Build history of the part. All positions in model axes, mm. Round coordinates to 2 decimals unless told otherwise and drop trailing zeros. Order: outer loops, then holes, each group sorted by start corner. A loop starts at its lowest first (then second) coordinate and runs counter-clockwise, first axis right, second up. Notation, with made-up numbers: (56.25, 4.5) -> (104.25, 4.5) arc R18 cw to (104.25, 22.5) -> close; hole circle Ø3 at (-1, 87.5). An arc over 180 degrees is marked (long way). Write item = value, one per line.
Autodesk Inventor part; units mm, degrees
ref_plane "工作平面1" through (0, 0, 0) normal (0, 0, 1) x (1, 0, 0)
ref_plane "工作平面2" through (173.2, -616.2, 0) normal (1, 0, 0) x (0, 0, -1)
ref_plane "工作平面3" through (318, -1163.6, 0) normal (1, 0, 0) x (0, 0, -1)
ref_plane "工作平面1" through (0, 0, 0) normal (0, 0, 1) x (1, 0, 0)
sketch "草图1" plane through (0, 0, 0) normal (0, 0, 1) x (1, 0, 0)
  line L0 (0, 0) -> (60, 0)
  line L1 (60, 0) -> (60, -1169.8)
  line L2 (60, -1169.8) -> (0, -1169.8)
  line L3 (0, -1169.8) -> (0, 0)
  line L4 (0, -80.6) -> (60, -80.6)
  line L5 (0, -191.9) -> (60, -191.9)
  line L6 (0, -276.5) -> (60, -276.5)
  line L7 (0, -335.9) -> (60, -335.9)
  line L8 (0, -420.6) -> (60, -420.6)
  line L9 (0, -550.6) -> (60, -550.6)
  line L10 (0, -677.8) -> (60, -677.8)
  line L11 (0, -782.9) -> (60, -782.9)
  line L12 (0, -839.5) -> (60, -839.5)
  line L13 (0, -923.6) -> (60, -923.6)
  line L14 (0, -1007.7) -> (60, -1007.7)
  line L15 (0, -1091.2) -> (60, -1091.2)
  line L16 (60, 0) -> (118.4, 0)
  line L17 (118.4, 0) -> (118.4, -23.7)
  line L18 (118.4, -23.7) -> (83.4, -23.7)
  line L19 (83.4, -23.7) -> (83.4, -79.7)
  line L20 (83.4, -79.7) -> (118.4, -79.7)
  line L21 (118.4, -79.7) -> (118.4, -137.6)
  line L22 (118.4, -137.6) -> (83.4, -137.6)
  line L23 (83.4, -137.6) -> (83.4, -276.5)
  line L24 (83.4, -276.5) -> (142.9, -276.5)
  line L25 (142.9, -276.5) -> (142.9, -379.5)
  line L26 (83.4, -276.5) -> (83.4, -379.5)
  line L27 (83.4, -379.5) -> (142.9, -379.5)
  line L28 (142.9, -379.5) -> (142.9, -463)
  line L29 (142.9, -463) -> (83.4, -463)
  line L30 (83.4, -463) -> (83.4, -379.5)
  line L31 (142.9, -463) -> (142.9, -566.2)
  line L32 (142.9, -566.2) -> (83.4, -566.2)
  line L33 (83.4, -566.2) -> (83.4, -463)
  line L34 (142.9, -566.2) -> (146.7, -566.2)
  line L35 (146.7, -566.2) -> (146.7, -616.2)
  line L36 (146.7, -616.2) -> (192.5, -616.2)
  line L37 (192.5, -616.2) -> (192.5, -673.2)
  line L38 (192.5, -616.2) -> (342.5, -616.2)
  line L39 (342.5, -616.2) -> (342.5, -673.2)
  line L40 (342.5, -673.2) -> (143.4, -673.2)
  line L41 (143.4, -673.2) -> (83.4, -673.2)
  line L42 (83.4, -673.2) -> (83.4, -1092.3)
  line L43 (83.4, -1092.3) -> (143.4, -1092.3)
  line L44 (143.4, -1092.3) -> (143.4, -673.2)
  line L45 (83.4, -754.3) -> (143.4, -754.3)
  line L46 (143.4, -837.8) -> (83.4, -837.8)
  line L47 (83.4, -893.6) -> (143.4, -893.6)
  line L48 (143.4, -978.3) -> (83.4, -978.3)
  line L49 (60, -1169.8) -> (188.1, -1169.8)
  line L50 (188.1, -1169.8) -> (188.1, -1092.3)
  line L51 (188.1, -1092.3) -> (143.4, -1092.3)
  line L52 (83.4, -1092.3) -> (83.4, -1117.3)
  line L53 (83.4, -1117.3) -> (188.1, -1117.3)
  line L54 (98.6, -1092.3) -> (98.6, -1117.3)
  line L55 (114.5, -1092.3) -> (114.5, -1117.3)
  line L56 (143.4, -1092.3) -> (143.4, -1117.3)
  line L57 (166.2, -1092.3) -> (166.2, -1117.3)
  line L58 (188.1, -1163.6) -> (336, -1163.6)
  line L59 (188.1, -1137.1) -> (336, -1137.1)
  line L60 (336, -1137.1) -> (336, -1163.6)
  dimension "d1" = 60
  dimension "d2" = 80.6
  dimension "d3" = 111.3
  dimension "d4" = 84.6
  dimension "d5" = 59.4
  dimension "d6" = 84.7
  dimension "d7" = 130
  dimension "d8" = 127.2
  dimension "d9" = 105.1
  dimension "d10" = 56.6
  dimension "d11" = 84.1
  dimension "d12" = 84.1
  dimension "d13" = 83.5
  dimension "d14" = 78.6
  dimension "d15" = 58.4
  dimension "d16" = 23.7
  dimension "d17" = 35
  dimension "d18" = 56
  dimension "d19" = 57.9
  dimension "d20" = 35
  dimension "d21" = 138.9
  dimension "d22" = 59.5
  dimension "d23" = 103
  dimension "d24" = 83.5
  dimension "d25" = 103.2
  dimension "d26" = 59.5
  dimension "d27" = 3.8
  dimension "d28" = 50
  dimension "d29" = 45.8
  dimension "d30" = 57
  dimension "d31" = 150
  dimension "d32" = 57
  dimension "d33" = 199.1
  dimension "d34" = 60
  dimension "d36" = 81.1
  dimension "d37" = 83.5
  dimension "d38" = 55.8
  dimension "d39" = 84.7
  dimension "d40" = 114
  dimension "d41" = 128.1
  dimension "d42" = 25
  dimension "d43" = 15.2
  dimension "d44" = 15.9
  dimension "d45" = 28.9
  dimension "d46" = 22.8
  dimension "d47" = 21.9
  dimension "d48" = 147.9
  dimension "d49" = 6.2
  dimension "d50" = 26.5
extrude "拉伸1" add sketch "草图1" against normal blind 1
sketch "草图2" plane through (0, 0, 0) normal (0, 0, 1) x (1, 0, 0)
  line L0 (342.5, -616.2) -> (146.7, -616.2) construction
  line L1 (342.5, -673.2) -> (342.5, -616.2) construction
  line L2 (143.4, -673.2) -> (342.5, -673.2) construction
  line L3 (146.7, -616.2) -> (146.7, -566.2) construction
  line L4 (150.3, -616.2) -> (150.3, -596.9)
  line L5 (150.3, -596.9) -> (196.1, -596.9)
  line L6 (196.1, -596.9) -> (196.1, -616.2)
  line L7 (150.3, -616.2) -> (196.1, -616.2)
  point P0 (0, 0)
  dimension "d53" = 19.3
  dimension "d54" = 45.8
  dimension "d55" = 3.6
extrude "拉伸2" add sketch "草图2" against normal up to surface (1 mm away)
ref_plane "工作平面2" through (173.2, -616.2, 0) normal (1, 0, 0) x (0, 0, -1)
sketch "草图3" plane through (173.2, -616.2, 0) normal (1, 0, 0) x (0, 0, -1)
  line L0 (0, 19.3) -> (1, 19.3) construction
  line L1 (0.5, 19.3) -> (-20.5, 61.3)
  line L2 (0.5, 19.3) -> (0.1, 19.3)
  line L3 (0.1, 19.3) -> (-20.9, 61.3)
  line L4 (-20.9, 61.3) -> (-20.5, 61.3)
  line L5 (-20.9, 61.3) -> (-20.9, 83.8)
  line L6 (-20.9, 83.8) -> (-20.5, 83.8)
  line L7 (-20.5, 83.8) -> (-20.5, 61.3)
  point P0 (0, 616.2)
  dimension "d58" = 42
  dimension "d60" = 21
  dimension "d61" = 0.4
  dimension "d64" = 22.5
extrude "拉伸3" add sketch "草图3" along normal up to surface (22.9 mm away)
extrude "拉伸4" add sketch "草图3" against normal up to surface (22.9 mm away) contours L4 L5 L6 L7
sketch "草图5" plane through (150.3, -554.9, 20.5) normal (-1, 0, 0) x (0, 0, 1)
  line L0 (0.4, 0) -> (0, 0) construction
  line L1 (0.2, 0) -> (21.2, -42) construction
  line L2 (0, 0) -> (21, -42)
  line L3 (0.4, 0) -> (0, 0)
  line L4 (0.4, 0) -> (21.4, -42)
  line L5 (21.4, -42) -> (21.2, -42)
  line L6 (21, -42) -> (21.2, -42)
  line L7 (21.4, -42) -> (21.4, -61.3)
  line L8 (21.4, -61.3) -> (21, -61.3)
  line L9 (21, -61.3) -> (21, -42)
  point P0 (-20.5, 554.9)
  dimension "d67" = 42
  dimension "d69" = 21
  dimension "d71" = 19.3
extrude "拉伸5" add sketch "草图5" against normal up to surface (22.9 mm away)
ref_plane "工作平面3" through (318, -1163.6, 0) normal (1, 0, 0) x (0, 0, -1)
sketch "草图6" plane through (318, -1163.6, 0) normal (1, 0, 0) x (0, 0, -1)
  line L0 (0, 26.5) -> (1, 26.5) construction
  line L1 (0.5, 26.5) -> (-20.5, 68.5)
  line L2 (0.5, 26.5) -> (0.1, 26.5)
  line L3 (0.1, 26.5) -> (-20.9, 68.5)
  line L4 (-20.9, 68.5) -> (-20.5, 68.5)
  line L5 (-20.9, 68.5) -> (-20.9, 93.5)
  line L6 (-20.9, 93.5) -> (-20.5, 93.5)
  line L7 (-20.5, 93.5) -> (-20.5, 68.5)
  point P0 (0, 1163.6)
  dimension "d75" = 42
  dimension "d77" = 21
  dimension "d78" = 0.4
  dimension "d79" = 25
  dimension "d80" = 0.4
extrude "拉伸6" add sketch "草图6" against normal blind 40
sketch "草图7" plane through (318, -1163.6, 0) normal (1, 0, 0) x (0, 0, -1)
  line L0 (-20.9, 93.5) -> (-20.9, 68.5) construction
  line L1 (-20.5, 68.5) -> (-20.5, 93.5) construction
  line L2 (-20.5, 93.5) -> (-20.9, 93.5) construction
  line L3 (-20.9, 93.5) -> (-20.5, 93.5)
  line L4 (-20.5, 93.5) -> (-20.5, 68.5)
  line L5 (-20.5, 68.5) -> (-20.9, 68.5)
  line L6 (-20.9, 68.5) -> (-20.9, 93.5)
  line L7 (-20.5, 68.5) -> (-41.5, 26.5)
  line L8 (-20.9, 68.5) -> (-41.9, 26.5)
  line L9 (-41.9, 26.5) -> (-41.5, 26.5)
  point P0 (0, 1163.6)
  dimension "d83" = 21
  dimension "d84" = 42
extrude "拉伸7" add sketch "草图7" along normal up to surface (18 mm away)
ref_plane "工作平面4" through (298, -1163.6, 0) normal (1, 0, 0) x (0, 0, -1)
mirror "镜像1" about plane through (298, -1163.6, 0) normal (1, 0, 0) of "拉伸7"
properties part number "LabVIEWM0.5"
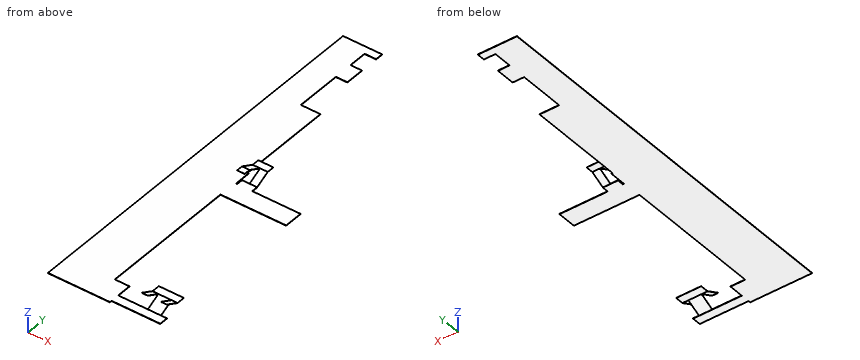
Q1. Cut at C-C, the plane y = -348.5. List the corners of the cut face in (x, z), and give its area (3 significant figures).
Check values:
outline = (0, -1) -> (142.9, -1) -> (142.9, 0) -> (0, 0) -> close
area = 143 mm²
Q2. Flat gauge pins, fed straight in: pin 1 (12 mm diameter, centred on x = 265.5, z = 33.5, fed in from +Y); pin 2 (1.1 mm diameter, centred on y = -1144.5, z = -0.5, fed in from +X); pin 3 (1.1 mm diameter, centred on x = 148.5, z = -0.5, fed in from +Y). Where does each tip first touch, or does it go through?
Check values:
pin_1 = -1108.3
pin_2 = 336
pin_3 = -616.2
Q3. Cut at A-A, the plane z = 28.5. List the corners of the cut face in (x, y), and give its area (3 significant figures).
Check values:
outline = (150.3, -570.9) -> (173.2, -570.9) -> (173.2, -570.1) -> (150.3, -570.1) -> close; (260, -1111.1) -> (278, -1111.1) -> (278, -1110.3) -> (260, -1110.3) -> close; (318, -1111.1) -> (336, -1111.1) -> (336, -1110.3) -> (318, -1110.3) -> close
area = 47.1 mm²
Q4. Probe probe 1 along Z at (x, y) = (125, -570); probe 2 along Y at (x, z) = (170.5, 30.5); probe 3 along Y at (x, z) = (318.5, 28). List the from-to ranges inside material, lowest first.
Check values:
probe_1 = -1 to 0
probe_2 = -574.9 to -574.1
probe_3 = -1110.1 to -1109.3
Q5. Cut at B-B, the plane x = 225.5. List the corners of the cut face in (y, z).
Check values:
outline = (-1163.6, -1) -> (-1137.1, -1) -> (-1137.1, 0) -> (-1163.6, 0) -> close; (-673.2, -1) -> (-616.2, -1) -> (-616.2, 0) -> (-673.2, 0) -> close
Q6. Cut at D-D, the plane y = -835. List the corners of the cut face in (x, z).
Check values:
outline = (0, -1) -> (143.4, -1) -> (143.4, 0) -> (0, 0) -> close
